For this review, take the finished solid that the model builds, in its own axes (mm). Give positions to 0.01 mm unless a question says otherwise; leave off trailing zeros. Order: outer loops, then holes, each group sorted by start corner. A loop starts at its lowest first (then second) coordinate and runs counter-clockwise, first axis right, second up.
Autodesk Inventor part; units mm, degrees
ref_plane "YZ Plane" through (0, 0, 0) normal (1, 0, 0) x (0, 1, 0)
ref_plane "XZ Plane" through (0, 0, 0) normal (0, 1, 0) x (-1, 0, 0)
ref_plane "XY Plane" through (0, 0, 0) normal (0, 0, 1) x (1, 0, 0)
sketch "Sketch1" plane through (0, 0, 0) normal (0, 0, 1) x (1, 0, 0)
  line L0 (0, 278.716) -> (197.082, 197.082) construction
  line L1 (197.082, 197.082) -> (278.716, 0) construction
  line L2 (278.716, 0) -> (197.082, -197.082) construction
  line L3 (197.082, -197.082) -> (0, -278.716) construction
  line L4 (0, -278.716) -> (-197.082, -197.082) construction
  line L5 (-197.082, -197.082) -> (-278.716, 0) construction
  line L6 (-278.716, 0) -> (-197.082, 197.082) construction
  line L7 (-197.082, 197.082) -> (0, 278.716)
  line L8 (-197.082, 197.082) -> (0, 278.716)
  line L9 (-461.6493, 774.8136) -> (-221.4406, 874.3113)
  line L10 (-98.541, 237.899) -> (-341.545, 824.5625) construction
  line L11 (-221.4406, 874.3113) -> (0, 874.3113)
  line L12 (0, 874.3113) -> (0, 278.716)
  line L13 (-461.6493, 774.8136) -> (-618.2315, 618.2315)
  line L14 (-618.2315, 618.2315) -> (-197.082, 197.082)
  point P0 (0, 0)
  point P1 (0, 0)
  dimension "d0" = 515
  dimension "d2" = 260
  dimension "d3" = 635
extrude "Extrusion1" add sketch "Sketch1" along normal mid plane 8
sketch "Sketch2" plane through (0, 0, 4) normal (0, 0, 1) x (1, 0, 0)
  line L0 (-221.4406, 874.3113) -> (-461.6493, 774.8136)
  line L1 (-461.6493, 774.8136) -> (-618.2315, 618.2315)
  line L2 (-236.7713, 532.4196) -> (-415.8262, 458.2526)
  line L3 (-197.082, 197.082) -> (0, 278.716)
  line L4 (-98.541, 237.899) -> (-341.545, 824.5625) construction
  line L5 (-618.2315, 618.2315) -> (-197.082, 197.082)
  line L6 (-415.8262, 458.2526) -> (-575.8051, 618.2315)
  line L7 (-575.8051, 618.2315) -> (-444.6557, 749.3809)
  line L8 (-444.6557, 749.3809) -> (-343.9227, 791.1058)
  line L9 (-236.7713, 532.4196) -> (-343.9227, 791.1058)
  line L10 (-209.0549, 543.9001) -> (-30, 618.067)
  line L11 (-30, 618.067) -> (-30, 844.3113)
  line L12 (-30, 844.3113) -> (-215.4733, 844.3113)
  line L13 (-215.4733, 844.3113) -> (-316.2063, 802.5863)
  line L14 (-209.0549, 543.9001) -> (-316.2063, 802.5863)
  line L15 (0, 278.716) -> (0, 874.3113)
  line L16 (-415.8262, 458.2526) -> (-30, 618.067) construction
  line L17 (-392.8652, 435.2916) -> (-30, 585.5953)
  line L18 (-190.043, 232.4694) -> (-30, 298.7614)
  line L19 (-30, 298.7614) -> (-30, 585.5953)
  line L20 (-190.043, 232.4694) -> (-392.8652, 435.2916)
  point P0 (0, 0)
  dimension "d11" = 30
  dimension "d12" = 280
  dimension "d13" = 30
  dimension "d14" = 30
  dimension "d15" = 15
  dimension "d21" = 30
  dimension "d22" = 30
  dimension "d23" = 30
  dimension "d24" = 30
extrude "Extrusion2" cut sketch "Sketch2" against normal up to surface (8 mm away)
fillet "Fillet1" radius 10 12 edges at (-575.8051, 618.2315, 0) (-343.9227, 791.1058, 0) (-236.7713, 532.4196, 0) (-415.8262, 458.2526, 0) (-316.2063, 802.5863, 0) (-30, 844.3113, 0) (-30, 618.067, 0) (-209.0549, 543.9001, 0) (-392.8652, 435.2916, 0) (-30, 585.5953, 0) (-30, 298.7614, 0) (-190.043, 232.4694, 0)
sketch "Sketch4" plane through (0, 0, 4) normal (0, 0, 1) x (1, 0, 0)
  line L0 (-221.4406, 874.3113) -> (-461.6493, 774.8136)
  line L1 (0, 874.3113) -> (-221.4406, 874.3113)
  line L2 (-461.6493, 774.8136) -> (-618.2315, 618.2315)
  line L3 (-618.2315, 618.2315) -> (-197.082, 197.082)
  line L4 (-197.082, 197.082) -> (0, 278.716)
  line L5 (0, 278.716) -> (0, 874.3113)
  line L6 (-458.817, 770.5748) -> (-220.4461, 869.3113)
  line L7 (-220.4461, 869.3113) -> (-5, 869.3113)
  line L8 (-5, 869.3113) -> (-5, 282.0569)
  line L9 (-5, 282.0569) -> (-195.9088, 202.9799)
  line L10 (-195.9088, 202.9799) -> (-611.1604, 618.2315)
  line L11 (-611.1604, 618.2315) -> (-458.817, 770.5748)
  line L12 (-218.8548, 861.3113) -> (-454.2854, 763.7928)
  line L13 (-454.2854, 763.7928) -> (-599.8467, 618.2315)
  line L14 (-599.8467, 618.2315) -> (-194.0317, 212.4165)
  line L15 (-194.0317, 212.4165) -> (-13, 287.4023)
  line L16 (-13, 287.4023) -> (-13, 861.3113)
  line L17 (-13, 861.3113) -> (-218.8548, 861.3113)
  point P0 (0, 0)
  dimension "d26" = 5
  dimension "d27" = 8
extrude "Extrusion3" cut sketch "Sketch4" against normal blind 3 contours L6 L7 L8 L9 L10 L11
fillet "Fillet3" radius 16 2 edges at (-220.4461, 869.3113, 2.5) (-458.817, 770.5748, 2.5)
fillet "Fillet4" radius 8 2 edges at (-454.2854, 763.7928, 2.5) (-218.8548, 861.3113, 2.5)
equation "\"d0\" = Барабан_размер_по_плоскостям"
equation "\"d2\" = Кассета_длина_грани"
equation "\"d3\" = Кассета_высота"
equation "\"d11\" = d13"
equation "\"d14\" = d13"
equation "\"d15\" = 0.5 * d13"
equation "\"d21\" = d13"
equation "\"d22\" = d13"
equation "\"d23\" = d13"
equation "\"d24\" = d13"
properties part number "DMF 01 51 outside frame v2.1"
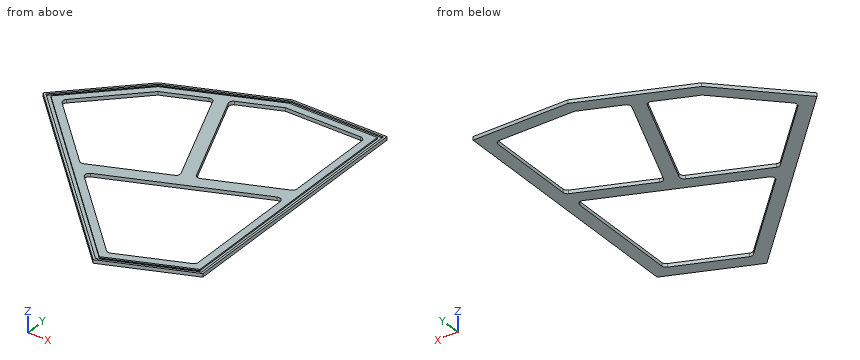
1) We need section D-D on y = 652. Give the boundary of the cut face in (x, z).
Answer sheet:
outline: (-584.46, -4) - (-542.04, -4) - (-542.04, 4) - (-566.08, 4) - (-566.08, 1) - (-577.39, 1) - (-577.39, 4) - (-584.46, 4) - close; (-286.3, -4) - (-253.83, -4) - (-253.83, 4) - (-286.3, 4) - close; (-30, -4) - (0, -4) - (0, 4) - (-5, 4) - (-5, 1) - (-13, 1) - (-13, 4) - (-30, 4) - close
2) To check wall thickness, follow line 1 (Y direction, x = -99.5, z = -3.25); line 2 (Y direction, x = -434.5, z = 1.5); line 3 (Y direction, x = -365.5, z = 0.25). State the ranges of each line that lie inside material, in increasing order.
Answer sheet:
line 1: y = 237.5 to 269.97, 556.81 to 589.28, 844.31 to 874.31
line 2: y = 434.5 to 441.57, 452.88 to 476.93, 753.59 to 771.99, 780.65 to 786.06
line 3: y = 365.5 to 407.93, 446.63 to 479.1, 782.17 to 814.64
3) Clearance check with flat-ended pins moving along their axes: pin 1 (2.5 mm diameter, centred on y = 424, z = -0.5, fed in from -X); pin 2 (2.5 mm diameter, centred on x = -99, z = 0, fed in from -Y); pin 3 (3.5 mm diameter, centred on y = 637.5, z = 2, fed in from -X). State where each tip first meets the part, or that it passes through.
Answer sheet:
pin 1: stops at x = -425.25
pin 2: stops at y = 237.19
pin 3: stops at x = -600.71
4) We need section C-C on y = 264.5. Give the boundary of the cut face in (x, z).
Answer sheet:
outline: (-264.5, -4) - (-222.07, -4) - (-222.07, 4) - (-246.12, 4) - (-246.12, 1) - (-257.43, 1) - (-257.43, 4) - (-264.5, 4) - close; (-112.71, -4) - (-34.32, -4) - (-34.32, 4) - (-47.39, 4) - (-47.39, 1) - (-68.29, 1) - (-68.29, 4) - (-112.71, 4) - close
5) We need section A-A on z = -1. Count the separate pieces of the cut face and the enclosed holes in it, then the cut area to 3 significant figures.
Answer sheet:
separate pieces: 1
enclosed holes: 3
area: 80,700 mm2
6) We need section B-B on x = -490.5. Give the boundary of the cut face in (y, z), then the cut area to 3 significant figures.
Answer sheet:
outline: (490.5, -4) - (532.93, -4) - (532.93, 4) - (508.88, 4) - (508.88, 1) - (497.57, 1) - (497.57, 4) - (490.5, 4) - close; (703.54, -4) - (745.96, -4) - (745.96, 4) - (738.89, 4) - (738.89, 1) - (727.58, 1) - (727.58, 4) - (703.54, 4) - close
area: 611 mm2
